Study the drawing (mm; zero at the part's minimum x, y, z) and answer. Coordinates: 2 decimals unless noted, no trailing zeros. Loops run counter-clockwise (first coordinate to the right, second up) from the corner with the lowest first, then second, coordinate; pieces in that order, holes last. Notation, with made-up numbers: (82, 77.25) -> (112, 77.25) arc R13 ccw to (112, 87.25) -> close; hole circle Ø2 at (81.25, 76). An arc over 180 degrees is marked (long way). One line per question, with ' | ' between items.
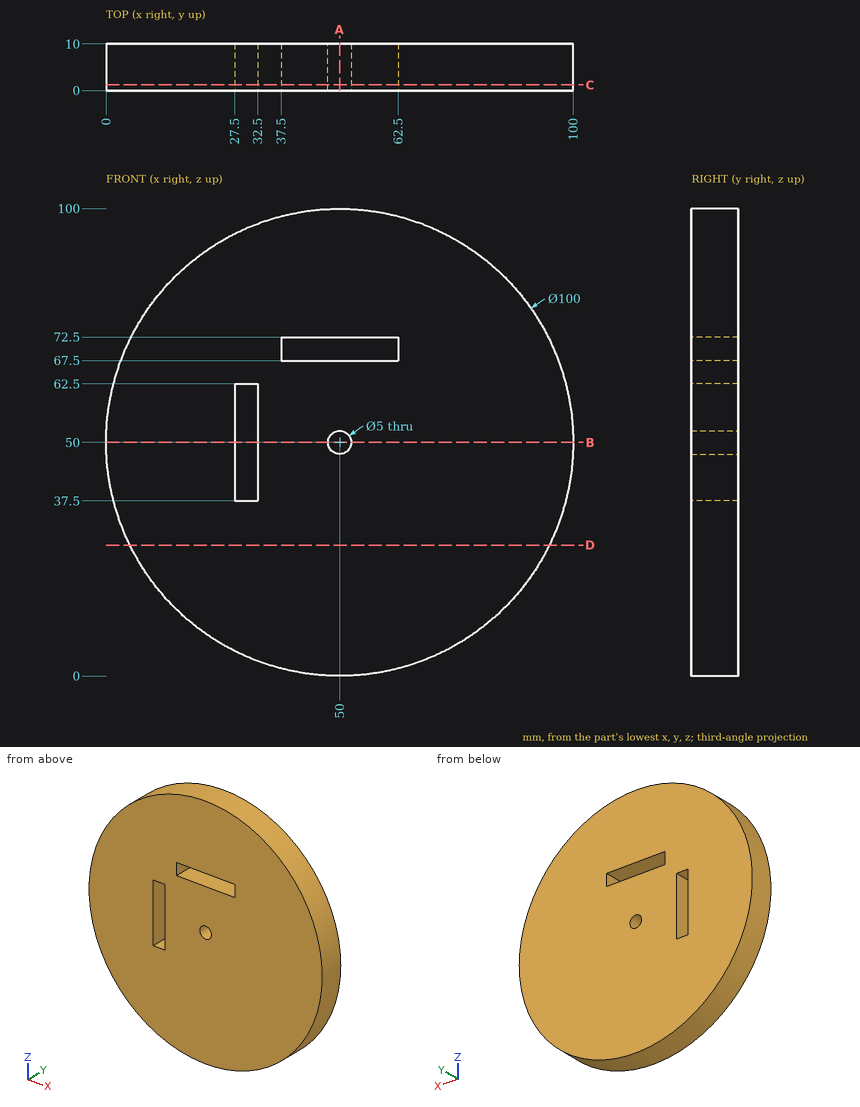
1) Find section D-D (z = 28). Write down the section's boundary in (x, y), plus the area to 3 significant figures.
Check values:
outline: (5.1, 0) -> (94.9, 0) -> (94.9, 10) -> (5.1, 10) -> close | area: 898 mm^2
2) Find the intervals of material crossed by line 1 along X through (y, z) = (2.5, 50); line 2 along Z through (x, y) = (50, 7.5); line 3 along Z through (x, y) = (30.5, 4.75), in increasing order.
Check values:
line 1: x = 0 to 27.5, 32.5 to 47.5, 52.5 to 100 | line 2: z = 0 to 47.5, 52.5 to 67.5, 72.5 to 100 | line 3: z = 3.96 to 37.5, 62.5 to 96.04
3) Find section A-A (x = 50). Write down the section's boundary in (y, z).
Check values:
outline: (0, 0) -> (10, 0) -> (10, 47.5) -> (0, 47.5) -> close; (0, 52.5) -> (10, 52.5) -> (10, 67.5) -> (0, 67.5) -> close; (0, 72.5) -> (10, 72.5) -> (10, 100) -> (0, 100) -> close
4) Flat-ended cylindrical pins translate along their axes: pin 1 (1.5 mm diameter, centred on y = 4, z = 69, fed in from -X); pin 2 (3 mm diameter, centred on x = 36, y = 4, fed in from -Z); pin 3 (5 mm diameter, centred on x = 45.5, y = 4, fed in from -Z). Find the tip coordinate at first contact, or state that the pin passes through.
Check values:
pin 1: stops at x = 3.45 | pin 2: stops at z = 1.59 | pin 3: stops at z = 0.04
5) Find section B-B (z = 50). Write down the section's boundary in (x, y), plus the area to 3 significant figures.
Check values:
outline: (0, 0) -> (27.5, 0) -> (27.5, 10) -> (0, 10) -> close; (32.5, 0) -> (47.5, 0) -> (47.5, 10) -> (32.5, 10) -> close; (52.5, 0) -> (100, 0) -> (100, 10) -> (52.5, 10) -> close | area: 900 mm^2
6) Find section C-C (y = 1.25). Write down the section's boundary in (x, z).
Check values:
outline: circle Ø100 at (50, 50); hole (27.5, 37.5) -> (32.5, 37.5) -> (32.5, 62.5) -> (27.5, 62.5) -> close; hole (37.5, 67.5) -> (62.5, 67.5) -> (62.5, 72.5) -> (37.5, 72.5) -> close; hole circle Ø5 at (50, 50)
